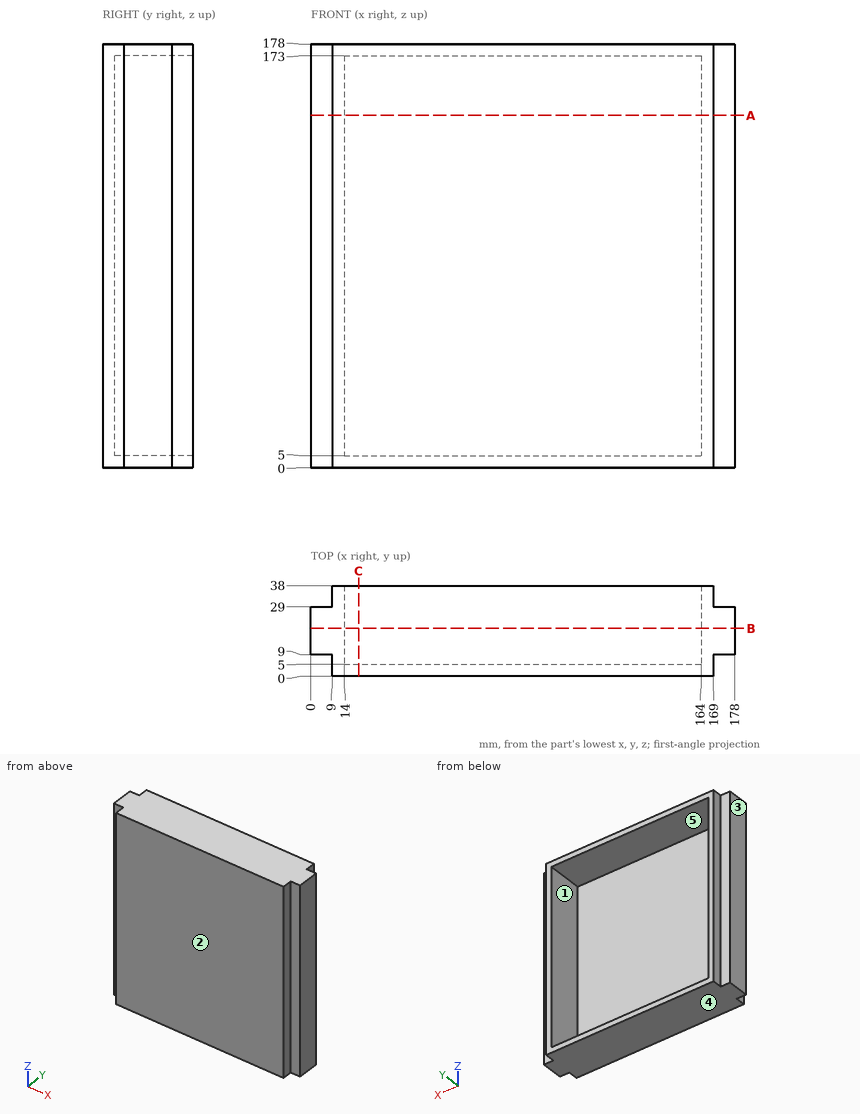
Input: dimensioned drawing with shaded views. Units: mm. Origin: part minimum x, y, z. A direction names the side the tool comes from. Coordinates: 2 decimals unless noted, no trailing zeros. Order: outer loops, then holes, each group sorted by start corner. A loop starts at its lowest first (then second) coordinate and runs counter-clockwise, first axis right, second up.
(1) Section query A-A (z = 148). Return the cut outline in (x, y).
(2) Section query C-C (x = 20). Return the cut outline in (y, z), plus the area to 3 significant figures.
(3) Section query B-B (y = 20). Return the cut outline in (x, z).
(4) Draft query along X for the marked faces 1, 2 and 3. Return one class per face: pulls with the +X half, pulls with the -X half, needs draft (parallel to the pull), parting line crosses it, or undercut.
(5) First-contact query: pin 1 (7 mm diameter, centred on y = 6.5, z = 83, fed in from +X); pin 2 (1.5 mm diameter, centred on x = 63, z = 32, fed in from +Y); pin 3 (4.5 mm diameter, centred on y = 34, z = 121, fed in from -X); pin 4 (4.5 mm diameter, centred on x = 173, z = 127.5, fed in from +Y). Flat tips, straight axial feed; report the tip coordinate or a pass-through.
(6) Material intervals for probe 1 along Z at (x, y) = (162.5, 11); probe 2 along X at (y, z) = (34, 139); probe 3 along X at (y, z) = (10.5, 35), sorted ascending.
(7) Access query for the marked faces 4 and 5. Directions: +Z, -Z, +X, -X, +Y, -Y. A direction counts if a zero-diameter tool reaches every point of the face in a straight line with its end or side. Return the directions, or none.
Solution:
1. outline: (0, 9) - (9, 9) - (9, 0) - (169, 0) - (169, 9) - (178, 9) - (178, 29) - (169, 29) - (169, 38) - (164, 38) - (164, 5) - (14, 5) - (14, 38) - (9, 38) - (9, 29) - (0, 29) - close
2. outline: (0, 0) - (38, 0) - (38, 5) - (5, 5) - (5, 173) - (38, 173) - (38, 178) - (0, 178) - close
2. area: 1,220 mm2
3. outline: (0, 0) - (178, 0) - (178, 178) - (0, 178) - close; hole (14, 5) - (164, 5) - (164, 173) - (14, 173) - close
4. face 1: undercut
4. face 2: needs draft
4. face 3: pulls with the -X half
5. pin 1: stops at x = 178
5. pin 2: stops at y = 5
5. pin 3: stops at x = 9
5. pin 4: stops at y = 29
6. probe 1: z = 0 to 5, 173 to 178
6. probe 2: x = 9 to 14, 164 to 169
6. probe 3: x = 0 to 14, 164 to 178
7. face 4: -Z, +X, -X, +Y, -Y
7. face 5: +Y
